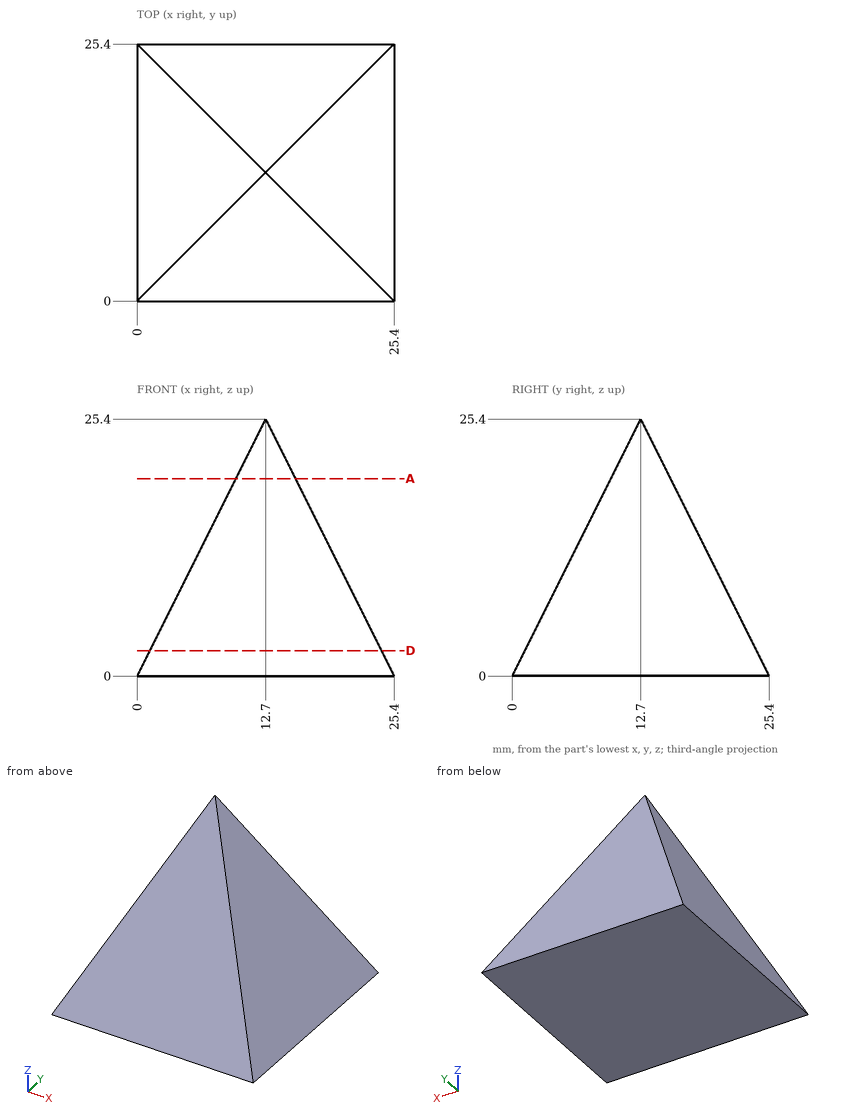
Verification items for this drawing (mm, ordinates from the low corner). Give positions to 0.01 mm unless a question says otherwise; leave off trailing zeros. Write each loop counter-clockwise with the first axis right and the second up, starting at its lowest first coordinate (ties: lowest second). Pieces come first, ordered by that corner, then holes. Notation, with made-up numbers: (42.5, 3) -> (49.5, 3) arc R23 cw to (49.5, 39) -> close; hole circle Ø5 at (64, 38). An arc over 180 degrees is marked (long way). Use CSV: the item, a comma, the result in double quotes. Start each with the question number.
Q1. Cross-section at A-A on z = 19.5. Enter the section's corners in (x, y).
Q2. Scan lines: line 1 along X through (y, z) = (6.25, 5.5); line 2 along Z through (x, y) = (12, 11); line 3 along Z through (x, y) = (21.5, 8.25). Record each from-to range of solid material in increasing order.
Q3. Depth check by flat-ended pin: P1, Ø1.5, axis at y = 8.5, z = 12.5, coming from the +X side (3 decimals); P2, Ø4, axis at y = 19.5, z = 3.5, coming from the -X side; P3, Ø10, axis at y = 6, z = 18.5, coming from the +X side; P4, Ø12, axis at y = 22.5, z = 22.5, coming from the +X side. Enter the tip coordinate at first touch or a pass-through.
Q4. Cross-section at D-D on z = 2.5. Enter the section's corners in (x, y).
Working result:
1,outline,"(9.75, 9.75) -> (15.65, 9.75) -> (15.65, 15.65) -> (9.75, 15.65) -> close"
2,line 1,"x = 2.75 to 22.65"
2,line 2,"z = 0 to 22"
2,line 3,"z = 0 to 7.8"
3,P1,"stops at x = 19.525"
3,P2,"stops at x = 0.75"
3,P3,"stops at x = 18.62"
3,P4,"passes through"
4,outline,"(1.25, 1.25) -> (24.15, 1.25) -> (24.15, 24.15) -> (1.25, 24.15) -> close"
